```python
from build123d import *

# Parameters (mm, degrees)
BOSS_EXTRUDE1_DEPTH = 266.7
SKETCH7_R           = 2.575
CUT_EXTRUDE5_DEPTH  = 270.426391849
SKETCH8_R           = 2.5
CUT_EXTRUDE7_DEPTH  = 270.426391849


with BuildPart() as part:
    # Sketch1 → Boss-Extrude1 (new body)
    with BuildSketch(Plane.XY):
        with BuildLine():
            Line((-12.7, 0), (12.7, 0))
            Line((12.7, 0), (12.7, 6.35))
            Line((12.7, 6.35), (12.7, 28.575))
            Line((12.7, 28.575), (11.049, 28.575))
            ThreePointArc((11.049, 28.575), (9.971369265, 28.128630735), (9.525, 27.051))
            Line((9.525, 27.051), (9.525, 4.699))
            ThreePointArc((9.525, 4.699), (9.078630735, 3.621369265), (8.001, 3.175))
            Line((8.001, 3.175), (-8.001, 3.175))
            ThreePointArc((-8.001, 3.175), (-9.078630735, 3.621369265), (-9.525, 4.699))
            Line((-9.525, 4.699), (-9.525, 27.051))
            ThreePointArc((-9.525, 27.051), (-9.971369265, 28.128630735), (-11.049, 28.575))
            Line((-11.049, 28.575), (-12.7, 28.575))
            Line((-12.7, 28.575), (-12.7, 3.175))
            Line((-12.7, 3.175), (-12.7, 0))
        make_face()
    extrude(amount=BOSS_EXTRUDE1_DEPTH)

    # Sketch7 → Cut-Extrude5 (cut, through all)
    with BuildSketch(Plane(origin=(12.7, 0, 0), x_dir=(0, 0, -1), z_dir=(1, 0, 0))):
        with Locations(Location((-216.108705962, 15.875, 0), (0, 0, 90))):
            Circle(SKETCH7_R)
        with Locations(Location((-249.836235321, 15.875, 0), (0, 0, 90))):
            Circle(SKETCH7_R)
    extrude(amount=-CUT_EXTRUDE5_DEPTH, mode=Mode.SUBTRACT)

    # Sketch8 → Cut-Extrude7 (cut, through all)
    with BuildSketch(Plane.ZY.offset(12.7)):
        with Locations((10.35, 15.875)):
            Circle(SKETCH8_R)
        with Locations((27.35, 15.875)):
            Circle(SKETCH8_R)
    extrude(amount=-CUT_EXTRUDE7_DEPTH, mode=Mode.SUBTRACT)


solid = part.part
```
Read the model definition and answer for the solid it produces. Units are mm, in the model's axes. A direction names the side the tool comes from. Coordinates: 2 decimals unless noted, no trailing zeros. Write each loop counter-clockwise with the first axis right and the second up, starting at its lowest first coordinate (ties: lowest second). Pieces come first, ordered by that corner, then holes. Notation, with made-up numbers: (18, -15.75) -> (73, -15.75) arc R14 ccw to (73, -8.75) -> close; hole circle Ø8 at (-6.75, 70.25). An arc over 180 degrees is marked (long way). Answer as a JSON object with one key per item and string values.
Q1. Determine the mould class of faces 3 (the flat face through (9.525, 16, 131)), 4 (the cylindrical face through (-11.13, 14.35, 8.37)), 5 (the flat face through (-12.7, 14, 131)) for opening direction X: pulls with the +X half, pulls with the -X half, needs draft (parallel to the pull), parting line crosses it, or undercut.
The answers:
{"face 3": "undercut", "face 4": "needs draft", "face 5": "pulls with the -X half"}
Q2. The part is cut by section C-C on z = 123. Give the vertices of the cut face in (x, y) (3 decimals), then the cut area to 3 significant figures.
The answers:
{"outline": "(-12.7, 0) -> (12.7, 0) -> (12.7, 28.575) -> (11.049, 28.575) arc R1.524 ccw to (9.525, 27.051) -> (9.525, 4.699) arc R1.524 cw to (8.001, 3.175) -> (-8.001, 3.175) arc R1.524 cw to (-9.525, 4.699) -> (-9.525, 27.051) arc R1.524 ccw to (-11.049, 28.575) -> (-12.7, 28.575) -> close", "area": "242 mm2"}
Q3. The part is cut by section D-D on x = 3. Give the vertices of the cut face in (y, z) (3 decimals).
The answers:
{"outline": "(0, 0) -> (3.175, 0) -> (3.175, 266.7) -> (0, 266.7) -> close"}
Q4. The part is cut by section B-B on z = 10.35. Give the vertices of the cut face in (x, y) (3 decimals).
The answers:
{"outline": "(-12.7, 0) -> (12.7, 0) -> (12.7, 13.375) -> (9.525, 13.375) -> (9.525, 4.699) arc R1.524 cw to (8.001, 3.175) -> (-8.001, 3.175) arc R1.524 cw to (-9.525, 4.699) -> (-9.525, 13.375) -> (-12.7, 13.375) -> close; (-12.7, 18.375) -> (-9.525, 18.375) -> (-9.525, 27.051) arc R1.524 ccw to (-11.049, 28.575) -> (-12.7, 28.575) -> close; (9.525, 18.375) -> (12.7, 18.375) -> (12.7, 28.575) -> (11.049, 28.575) arc R1.524 ccw to (9.525, 27.051) -> close"}
Q5. A tool of negligible diameter and unlimited length cuts with its end or side. For faces 1 (the flat face through (-9.525, 16, 131)), 2 (the flat face through (12.7, 14, 131)), from which of +Z, -Z, +X, -X, +Y, -Y can it reach the whole face along a straight path? Write none if from no direction.
The answers:
{"face 1": "+Z, -Z, +Y", "face 2": "+Z, -Z, +X, +Y, -Y"}
Q6. Consider line 1 (X direction, y = 7.25, z = 52.5) (3 decimals); line 2 (Y direction, x = 11.45, z = 10.35) (3 decimals); line 3 (Y direction, x = -4.75, z = 124.5) (3 decimals). Determine where each line is inside the solid, lowest interval first. Write a range as [from, to].
The answers:
{"line 1": "x = [-12.7, -9.525], [9.525, 12.7]", "line 2": "y = [0, 13.375], [18.375, 28.575]", "line 3": "y = [0, 3.175]"}
Q7. Flat-ended cylindrical pins translate along their axes: pin 1 Ø6 at (y, z) = (15.88, 249.84) entering from -X; pin 2 Ø3 at (y, z) = (15.875, 27.35) entering from -X; pin 3 Ø1 at (x, z) = (1, 109.5) entering from +Y (3 decimals); pin 4 Ø12 at (x, z) = (3, 194) entering from +Y. Find the tip coordinate at first contact, or state that the pin passes through.
The answers:
{"pin 1": "stops at x = -12.7", "pin 2": "passes through", "pin 3": "stops at y = 3.175", "pin 4": "stops at y = 3.55"}
Q8. The part is cut by section A-A on y = 9.25. Give the vertices of the cut face in (x, z) (3 decimals).
The answers:
{"outline": "(-12.7, 0) -> (-9.525, 0) -> (-9.525, 266.7) -> (-12.7, 266.7) -> close; (9.525, 0) -> (12.7, 0) -> (12.7, 266.7) -> (9.525, 266.7) -> close"}
